```python
from build123d import *

# Parameters (mm, degrees)
F1_R     = 10.2
F1_R_2   = 8.85
F2_DEPTH = 2
F1_R_3   = 12
F1_R_4   = 7.5
F3_DEPTH = 2.5


with BuildPart() as f2:
    # F1 (on Front) → F2 (new body, symmetric)
    with BuildSketch(Plane.XZ):
        Circle(F1_R)
        Circle(F1_R_2, mode=Mode.SUBTRACT)
    extrude(amount=F2_DEPTH, both=True)

    # F1 (on Front) → F3 (join, symmetric)
    with BuildSketch(Plane.XZ):
        Circle(F1_R_3)
        Circle(F1_R, mode=Mode.SUBTRACT)
        Circle(F1_R_2)
        Circle(F1_R_4, mode=Mode.SUBTRACT)
    extrude(amount=F3_DEPTH, both=True)


solid = f2.part
```
For this review, take the finished solid that the model builds, in its own axes (mm). A direction names the side the tool comes from. Round coordinates to 2 decimals unless told otherwise and drop trailing zeros. Loops run counter-clockwise (first coordinate to the right, second up) from the corner with the lowest first, then second, coordinate; pieces in that order, holes last.
(1) We need section B-B (z = 0). Give the boundary of the cut face in (x, y), plus the area to 3 significant figures.
Returned:
outline: (-12, -2.5) - (-10.2, -2.5) - (-10.2, -2) - (-8.85, -2) - (-8.85, -2.5) - (-7.5, -2.5) - (-7.5, 2.5) - (-8.85, 2.5) - (-8.85, 2) - (-10.2, 2) - (-10.2, 2.5) - (-12, 2.5) - close; (7.5, -2.5) - (8.85, -2.5) - (8.85, -2) - (10.2, -2) - (10.2, -2.5) - (12, -2.5) - (12, 2.5) - (10.2, 2.5) - (10.2, 2) - (8.85, 2) - (8.85, 2.5) - (7.5, 2.5) - close
area: 42.3 mm2
(2) We need section D-D (x = -9.5). Give the boundary of the cut face in (y, z).
Returned:
outline: (-2.5, -7.33) - (2.5, -7.33) - (2.5, -3.71) - (2, -3.71) - (2, 3.71) - (2.5, 3.71) - (2.5, 7.33) - (-2.5, 7.33) - (-2.5, 3.71) - (-2, 3.71) - (-2, -3.71) - (-2.5, -3.71) - close
(3) Tool access review of faces 1 (the cylindrical face through (8.44, -2.25, 2.66)), 2 (the cylindrical face through (8.44, 2.25, 2.66)), 3 (the cylindrical face through (-7.493, 0.035, 0.33)): name each direction out of +Z, -Z, +X, -X, +Y, -Y from which nothing blocks a thin tool from reaching the whole face with its end or side.
Returned:
face 1: -Y
face 2: +Y
face 3: +Y, -Y
(4) Clearance check with flat-ended pins moving along their axes: P1, Ø13.5, axis at x = 0, z = 0, coming from the +Y side; P2, Ø4, axis at x = 5.5, z = -3, coming from the -Y side; P3, Ø3, axis at y = -1, z = -2.5, coming from the -X side; P4, Ø3, axis at y = 0, z = 2, coming from the +X side. State where each tip first meets the part, or that it passes through.
Returned:
P1: passes through
P2: stops at y = -2.5
P3: stops at x = -11.96
P4: stops at x = 11.99
(5) Wall thickness on line 1 along Z through (x, y) = (0, 2.25); line 2 along Z through (x, y) = (0, -1.3); line 3 along Y through (x, z) = (-9, 3): over which ranges is each line inside the solid? List them lowest first.
Returned:
line 1: z = -12 to -10.2, -8.85 to -7.5, 7.5 to 8.85, 10.2 to 12
line 2: z = -12 to -7.5, 7.5 to 12
line 3: y = -2 to 2
(6) Mouldability with a two-part tool opening along Z and no side actions: class faces 4 (the flat face through (-8, -2, 5)), 5 (the cylindrical face through (-11.99, -0.04, 0.53)), 6 (the flat face through (-4, 2.5, -10)) as released by +Z, released by -Z, zero draft, split by the parting line, or undercut.
Returned:
face 4: undercut
face 5: split by the parting line
face 6: zero draft
(7) We need section C-C (y = 1.1). Give the boundary of the cut face in (x, z), plus the area to 3 significant figures.
Returned:
outline: circle Ø24 at (0, 0); hole circle Ø15 at (0, 0)
area: 276 mm2
(8) We need section A-A (x = 0). Give the boundary of the cut face in (y, z), plus the area to 3 significant figures.
Returned:
outline: (-2.5, -12) - (2.5, -12) - (2.5, -10.2) - (2, -10.2) - (2, -8.85) - (2.5, -8.85) - (2.5, -7.5) - (-2.5, -7.5) - (-2.5, -8.85) - (-2, -8.85) - (-2, -10.2) - (-2.5, -10.2) - close; (-2.5, 7.5) - (2.5, 7.5) - (2.5, 8.85) - (2, 8.85) - (2, 10.2) - (2.5, 10.2) - (2.5, 12) - (-2.5, 12) - (-2.5, 10.2) - (-2, 10.2) - (-2, 8.85) - (-2.5, 8.85) - close
area: 42.3 mm2
